Print and shaded views of the part. All mm, measured from the part's lowest x, y and z. Round coordinates to 2 decimals unless told otherwise and drop trailing zeros. Order: outer loops, then holes, each group sorted by start corner. A loop starts at its lowest first (then second) coordinate and runs counter-clockwise, first axis right, second up. Notation, with made-up numbers: (43, 56.25) - (79, 56.25) arc R16 ccw to (79, 86.25) - close; hole circle Ø4 at (87.25, 37.25). An arc over 180 degrees is marked (long way). Return JSON: item names as keys, results as strings. Group by question number.
Item 1: Saw through at B-B on x = 109. List the corners of the cut face in (y, z).
Item 2: Drop flat-ended pins along their axis: pin 1 (3 mm diameter, centred on y = 3.5, z = 79.5, fed in from +X); pin 2 (8 mm diameter, centred on x = 19, z = 107, fed in from +Y) (3 decimals). Give the stop position or say it passes through.
Item 3: Saw through at A-A on z = 28. List the corners of the cut face in (x, y), and give its area (3 significant figures).
Item 4: Saw through at D-D on z = 56. List the corners of the cut face in (x, y), and give its area (3 significant figures).
Item 5: Probe probe 1 along X at (y, z) = (5.75, 105.5); probe 2 along Z at (x, y) = (75.5, 5.75); probe 3 along Z at (x, y) = (118, 5.75). List the from-to ranges inside material, lowest first.
Item 6: Saw through at C-C on y = 3. List the corners of the cut face in (x, z), and give its area (3 significant figures).
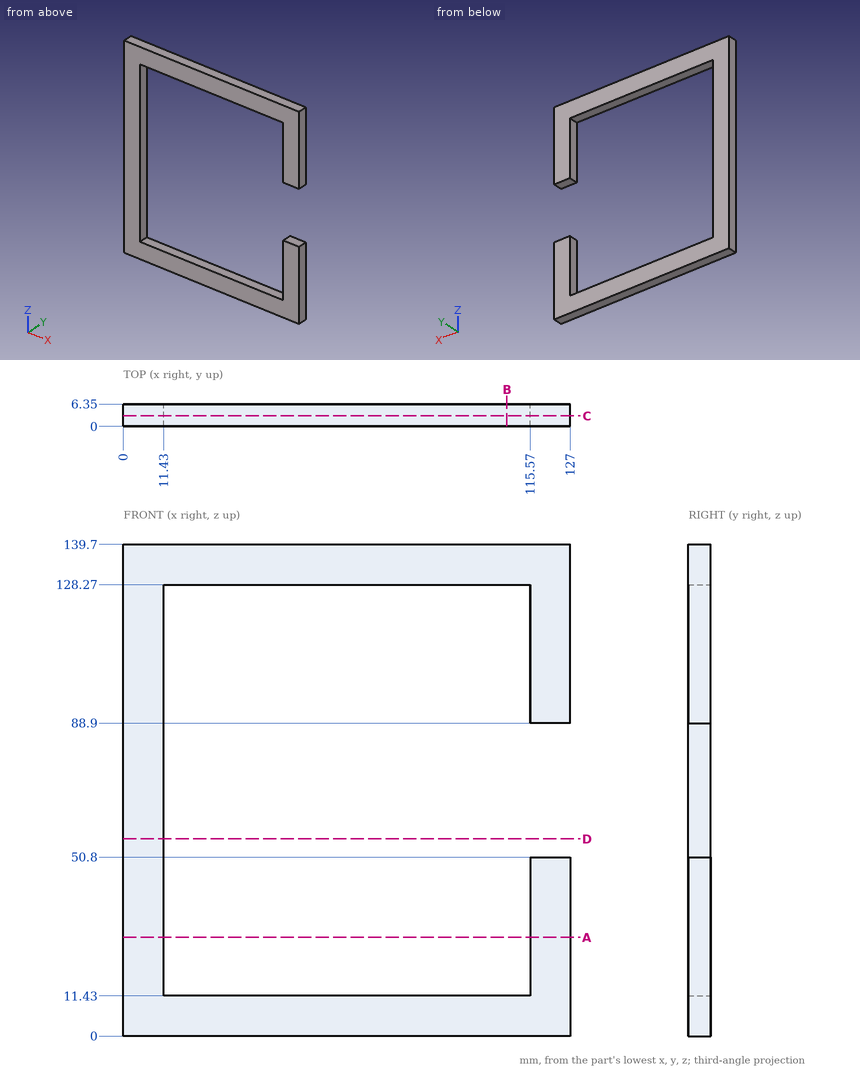
Filled in:
{
 "1": {"outline": "(0, 0) - (6.35, 0) - (6.35, 11.43) - (0, 11.43) - close; (0, 128.27) - (6.35, 128.27) - (6.35, 139.7) - (0, 139.7) - close"},
 "2": {"pin 1": "stops at x = 11.43", "pin 2": "passes through"},
 "3": {"outline": "(0, 0) - (11.43, 0) - (11.43, 6.35) - (0, 6.35) - close; (115.57, 0) - (127, 0) - (127, 6.35) - (115.57, 6.35) - close", "area": "145 mm^2"},
 "4": {"outline": "(0, 0) - (11.43, 0) - (11.43, 6.35) - (0, 6.35) - close", "area": "72.6 mm^2"},
 "5": {"probe 1": "x = 0 to 11.43, 115.57 to 127", "probe 2": "z = 0 to 11.43, 128.27 to 139.7", "probe 3": "z = 0 to 50.8, 88.9 to 139.7"},
 "6": {"outline": "(0, 0) - (127, 0) - (127, 50.8) - (115.57, 50.8) - (115.57, 11.43) - (11.43, 11.43) - (11.43, 128.27) - (115.57, 128.27) - (115.57, 88.9) - (127, 88.9) - (127, 139.7) - (0, 139.7) - close", "area": "5,140 mm^2"}
}
